from build123d import *

# Parameters (mm, degrees)
F0_W           = 10
F0_H           = 20
F1_DEPTH       = 10
F0_W_2         = 23
F2_DEPTH       = 8
F3_D           = 4.2
F4_D           = 4.5
F4_CBORE_D     = 8.25
F4_CBORE_DEPTH = 4


with BuildPart() as f1:
    # F0 (on Top) → F1 (new body)
    with BuildSketch(Plane.XY):
        with Locations((-11.5, 0)):
            Rectangle(F0_W, F0_H)
    extrude(amount=-F1_DEPTH)

    # F0 (on Top) → F2 (join)
    with BuildSketch(Plane.XY):
        with Locations((5, 0)):
            Rectangle(F0_W_2, F0_H)
    extrude(amount=-F2_DEPTH)

    # F3 (through all)
    with Locations(Plane.XY):
        with Locations((11.5, 0)):
            Hole(F3_D / 2)

    # F4 (through all)
    with Locations(Plane.XY):
        with Locations((-11.5, 5), (-11.5, -5)):
            CounterBoreHole(F4_D / 2, F4_CBORE_D / 2, F4_CBORE_DEPTH)


solid = f1.part
Read the model definition and answer for the solid it produces. Units are mm, in the model's axes. A direction names the side the tool comes from. Round coordinates to 2 decimals unless told otherwise and drop trailing zeros. Order: outer loops, then holes, each group sorted by start corner. A loop starts at its lowest first (then second) coordinate and runs counter-clockwise, first axis right, second up. Notation, with made-up numbers: (84.25, 7) - (138.25, 7) arc R22 ccw to (138.25, 40) - close; hole circle Ø10 at (22.25, 43). An arc over 180 degrees is marked (long way). Use one line per item in the form item = value. Start each with the question number.
(1) The part is cut by section C-C (z = -5.25). Give the vertices of the cut face in (x, y), then the cut area to 3 significant figures.
(2) The part is cut by section D-D (x = -11.5). Give the vertices of the cut face in (y, z) (3 decimals).
(3) The part is cut by section B-B (x = 11.5). Give the vertices of the cut face in (y, z).
(4) Find the intervals of material crossed by line 1 along Y through (x, z) = (-11.5, -2.25) (3 decimals); line 2 along Y through (x, z) = (-11.5, -5.4); line 3 along Y through (x, z) = (11.5, -2.25), in increasing order. Write a range as from..to.
(5) The part is cut by section A-A (y = 5). Give the vertices of the cut face in (x, z) (3 decimals).
(6) For faces 1 (the face through (0, 10, -4)), 2 (the face through (5, 0, -8)), 3 (the face through (-15.62, 5.18, -1.97)), determine the directions among +Z, -Z, +X, -X, +Y, -Y from which every point of the face is accessible in a straight line to the end or side of a thin tool.
(7) Determine the mould class of faces 4 (the face through (-15.62, -4.82, -1.97)), 5 (the face through (0, -10, -4)), 6 (the face through (-6.5, 0, -9)) for opening direction X: +X half, -X half, draft (parallel to the pull), parting line (faces both ways), or undercut.
(8) Flat-ended cylindrical pins translate along their axes: pin 1 Ø2.5 at (x, y) = (-12.5, -4) entering from +Z; pin 2 Ø1.6 at (y, z) = (1, -9.5) entering from +X; pin 3 Ø4 at (x, y) = (-11.5, 5) entering from +Z. Find the tip coordinate at first contact, or state that the pin passes through.
Checked values:
q1.outline = (-16.5, -10) - (16.5, -10) - (16.5, 10) - (-16.5, 10) - close; hole circle Ø4.5 at (-11.5, -5); hole circle Ø4.5 at (-11.5, 5); hole circle Ø4.2 at (11.5, 0)
q1.area = 614 mm^2
q2.outline = (-10, -10) - (-7.25, -10) - (-7.25, -4) - (-9.125, -4) - (-9.125, 0) - (-10, 0) - close; (-2.75, -10) - (2.75, -10) - (2.75, -4) - (0.875, -4) - (0.875, 0) - (-0.875, 0) - (-0.875, -4) - (-2.75, -4) - close; (7.25, -10) - (10, -10) - (10, 0) - (9.125, 0) - (9.125, -4) - (7.25, -4) - close
q3.outline = (-10, -8) - (-2.1, -8) - (-2.1, 0) - (-10, 0) - close; (2.1, -8) - (10, -8) - (10, 0) - (2.1, 0) - close
q4.line_1 = -10..-9.125, -0.875..0.875, 9.125..10
q4.line_2 = -10..-7.25, -2.75..2.75, 7.25..10
q4.line_3 = -10..-2.1, 2.1..10
q5.outline = (-16.5, -10) - (-13.75, -10) - (-13.75, -4) - (-15.625, -4) - (-15.625, 0) - (-16.5, 0) - close; (-9.25, -10) - (-6.5, -10) - (-6.5, -8) - (16.5, -8) - (16.5, 0) - (-7.375, 0) - (-7.375, -4) - (-9.25, -4) - close
q6.face_1 = +Z, -Z, +X, -X, +Y
q6.face_2 = -Z, +X, +Y, -Y
q6.face_3 = +Z
q7.face_4 = undercut
q7.face_5 = draft
q7.face_6 = +X half
q8.pin_1 = -4
q8.pin_2 = -6.5
q8.pin_3 = through
